Check sheet for the modelled part. Datum: model origin and axes. Units: mm. A direction names the side the tool comes from. Round coordinates to 2 decimals unless told otherwise and drop trailing zeros. Write each loop counter-clockwise with the first axis right and the second up, starting at its lowest first coordinate (ties: lowest second). Pieces come first, ordered by that corner, then holes. Notation, with made-up numbers: M 13.5,53 L 48.5,53 A25 cw 48.5,68 Z; hole C 87,88.25 d5. An arc over 180 degrees is marked long. One line per item, written item: value.
from build123d import *

# Parameters (mm, degrees)
BOSS_EXTRUDE1_DEPTH = 50.8
SKETCH2_R           = 1.7399
CUT_EXTRUDE1_DEPTH  = 45.72
FILLET1_R           = 2.54
SKETCH11_R          = 3.175
CUT_EXTRUDE5_DEPTH  = 2.54
SKETCH12_R          = 5.08
CUT_EXTRUDE6_DEPTH  = 72.906677743


with BuildPart() as part:
    # Sketch1 → Boss-Extrude1 (new body)
    with BuildSketch(Plane.XY):
        Polygon((0, 0), (0, -22.352), (10.16, -22.352), (10.16, -9.652), (45.72, -9.652), (45.72, 0), align=None)
    extrude(amount=BOSS_EXTRUDE1_DEPTH)

    # Sketch2 → Cut-Extrude1 (cut)
    with BuildSketch(Plane.ZY):
        with Locations(Location((4.3, -15.24, 0), (0, 0, 270))):
            Circle(SKETCH2_R)
        with Locations(Location((46.5, -15.24, 0), (0, 0, 270))):
            Circle(SKETCH2_R)
    extrude(amount=-CUT_EXTRUDE1_DEPTH, mode=Mode.SUBTRACT)

    # Fillet1
    fillet1_edges = [part.edges().sort_by_distance(p)[0] for p in [
        (10.16, -9.652, 25.4),
    ]]
    fillet(fillet1_edges, radius=FILLET1_R)

    # Sketch11 → Cut-Extrude5 (cut)
    with BuildSketch(Plane(origin=(10.16, 0, 0), x_dir=(0, 0, -1), z_dir=(1, 0, 0))):
        with Locations(Location((-46.5, -15.24, 0), (0, 0, 90))):
            Circle(SKETCH11_R)
        with Locations(Location((-4.3, -15.24, 0), (0, 0, 106.260204708))):
            Circle(SKETCH11_R)
    extrude(amount=-CUT_EXTRUDE5_DEPTH, mode=Mode.SUBTRACT)

    # Sketch12 → Cut-Extrude6 (cut, through all)
    with BuildSketch(Plane(origin=(0, 0, 0), x_dir=(1, 0, 0), z_dir=(0, 1, 0))):
        with Locations(Location((27.94, -27.94, 0), (0, 0, 270))):
            Circle(SKETCH12_R)
    extrude(amount=-CUT_EXTRUDE6_DEPTH, mode=Mode.SUBTRACT)


solid = part.part
Q1. Depth check by flat-ended pin: P1, Ø10, axis at x = 22.5, z = 25.5, coming from the -Y side; P2, Ø4.5, axis at y = -15.24, z = 4.3, coming from the -X side; P3, Ø5.5, axis at y = -15.24, z = 4.3, coming from the +X side; P4, Ø5, axis at y = -16.5, z = 31.5, coming from the +X side. Enter the tip coordinate at first touch or a pass-through.
Completed:
P1: y = -9.65
P2: x = 0
P3: x = 7.62
P4: x = 10.16
Q2. Sectioned sample at B-B on z = 27.94. Enter the section's corners in (x, y).
Completed:
outline: M 0,-22.35 L 10.16,-22.35 L 10.16,-12.19 A2.54 cw 12.7,-9.65 L 22.86,-9.65 L 22.86,0 L 0,0 Z; M 33.02,-9.65 L 45.72,-9.65 L 45.72,0 L 33.02,0 Z
Q3. Sectioned sample at D-D on z = 4.3. Enter the section's corners in (x, y) (3 decimals).
Completed:
outline: M 0,-22.352 L 10.16,-22.352 L 10.16,-18.415 L 7.62,-18.415 L 7.62,-16.98 L 0,-16.98 Z; M 0,-13.5 L 7.62,-13.5 L 7.62,-12.065 L 10.16,-12.065 L 10.16,-12.192 A2.54 cw 12.7,-9.652 L 45.72,-9.652 L 45.72,0 L 0,0 Z
Q4. Sectioned sample at A-A on x = 27.94. Enter the section's corners in (y, z).
Completed:
outline: M -9.65,0 L 0,0 L 0,22.86 L -9.65,22.86 Z; M -9.65,33.02 L 0,33.02 L 0,50.8 L -9.65,50.8 Z
Q5. Access from +Z, -Z, +X, -X, +Y, -Y to the whole of each face (thin tool, end or side, straight path). Record for faces 1 (the flat face through (33, -9.652, 25)), 2 (the flat face through (5, -22.352, 25)).
Completed:
face 1: +Z, -Z, +X, -Y
face 2: +Z, -Z, +X, -X, -Y
Q6. Sectioned sample at C-C on y = -15.24. Enter the section's corners in (x, z) (3 decimals), and give its area (3 significant figures).
Completed:
outline: M 0,0 L 10.16,0 L 10.16,1.125 L 7.62,1.125 L 7.62,2.56 L 0,2.56 Z; M 0,6.04 L 7.62,6.04 L 7.62,7.475 L 10.16,7.475 L 10.16,43.325 L 7.62,43.325 L 7.62,44.76 L 0,44.76 Z; M 0,48.24 L 7.62,48.24 L 7.62,49.675 L 10.16,49.675 L 10.16,50.8 L 0,50.8 Z
area: 431 mm^2
Q7. Draft check along Z on faces 3 (the flat face through (17, -6, 0)), 4 (the cylindrical face through (10.9, -10.4, 25.8)), 5 (the flat face through (7.62, -13.5, 3.4)). Enter one of: pulls with the +Z half, pulls with the -Z half, needs draft (parallel to the pull), parting line crosses it, or undercut.
Completed:
face 3: pulls with the -Z half
face 4: needs draft
face 5: undercut
Q8. Scan lines: line 1 (Z direction, x = 9.2, y = -15.24) (3 decimals); line 2 (Z direction, x = 3.5, y = -15.24); line 3 (Y direction, x = 9, z = 4). Record each from-to range of solid material in increasing order. Write a range as [from, to].
Completed:
line 1: [0, 1.125], [7.475, 43.325], [49.675, 50.8]
line 2: [0, 2.56], [6.04, 44.76], [48.24, 50.8]
line 3: [-22.35, -18.4], [-12.08, 0]
